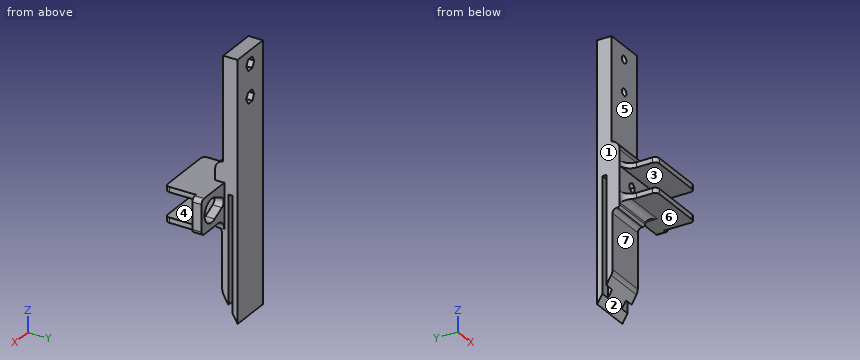
from build123d import *

# Parameters (mm, degrees)
SKETCH1_W                = 20
SKETCH1_H                = 8
BOSS_EXTRUDE1_DEPTH      = 125
CUT_EXTRUDE1_DEPTH       = 60
SKETCH3_W                = 20
SKETCH3_H                = 125
BOSS_EXTRUDE2_DEPTH      = 3
SKETCH5_W                = 4.5
SKETCH5_H                = 2
CUT_EXTRUDE2_DEPTH       = 60
BOSS_EXTRUDE5_DEPTH      = 15
BOSS_EXTRUDE5_DEPTH_BACK = 15
SKETCH9_W                = 2.5
SKETCH9_H                = 15
SKETCH10_W               = 17
SKETCH10_H               = 4.5
BOSS_EXTRUDE6_DEPTH      = 18
CUT_EXTRUDE3_DEPTH       = 129.663032374
CUT_EXTRUDE4_DEPTH       = 4
FILLET1_R                = 5
FILLET2_R                = 3
FILLET3_R                = 5
FILLET4_R                = 2
SKETCH13_W               = 46.736094472
SKETCH13_H               = 46.819354585
CUT_EXTRUDE5_DEPTH       = 30
SKETCH14_W               = 30.537207939
SKETCH14_H               = 50.61246041
CUT_EXTRUDE6_DEPTH       = 3.5
FILLET5_R                = 5
FILLET6_R                = 2
FILLET7_R                = 1
FILLET8_R                = 2
SKETCH15_W               = 20
SKETCH15_H               = 60
CUT_EXTRUDE7_DEPTH       = 5
SKETCH16_W               = 20
SKETCH16_H               = 60
BOSS_EXTRUDE7_DEPTH      = 1.5
SKETCH17_W               = 20
SKETCH17_H               = 10
BOSS_EXTRUDE8_DEPTH      = 4
FILLET9_R                = 5
SKETCH18_R               = 1.75
CUT_EXTRUDE8_DEPTH       = 131.403895283
CUT_EXTRUDE9_DEPTH       = 4


# Some blends are built 0.0001 mm under size
with BuildPart() as part:
    # Sketch1 → Boss-Extrude1 (new body)
    with BuildSketch(Plane.XY):
        with Locations((-16.536312849, 6.223463687)):
            Rectangle(SKETCH1_W, SKETCH1_H)
    extrude(amount=-BOSS_EXTRUDE1_DEPTH)

    # Sketch2 → Cut-Extrude1 (cut)
    with BuildSketch(Plane.XY):
        Polygon((-26.536312849, 7.723463687), (-22.186312849, 7.723463687), (-22.186312849, 5.723463687), (-23.686312849, 5.723463687), (-23.686312849, 4.223463687), (-22.186312849, 4.223463687), (-22.186312849, 2.723463687), (-20.536312849, 2.723463687), (-20.536312849, 7.723463687), (-12.536312849, 7.723463687), (-12.536312849, 2.723463687), (-10.886312849, 2.723463687), (-10.886312849, 4.223463687), (-9.386312849, 4.223463687), (-9.386312849, 5.723463687), (-10.886312849, 5.723463687), (-10.886312849, 7.723463687), (-6.536312849, 7.723463687), (-6.536312849, 2.223463687), (-26.536312849, 2.223463687), align=None)
    extrude(amount=-CUT_EXTRUDE1_DEPTH, mode=Mode.SUBTRACT)

    # Sketch3 → Boss-Extrude2 (add)
    with BuildSketch(Plane(origin=(0, 10.223463687, 0), x_dir=(1, 0, 0), z_dir=(0, 1, 0))):
        with Locations((-16.536312849, 62.5)):
            Rectangle(SKETCH3_W, SKETCH3_H)
    extrude(amount=BOSS_EXTRUDE2_DEPTH)

    # Sketch5 → Cut-Extrude2 (cut)
    with BuildSketch(Plane(origin=(0, 0, -125), x_dir=(-1, 0, 0), z_dir=(0, 0, -1))):
        with Locations((8.786312849, 9.723463687)):
            Rectangle(SKETCH5_W, SKETCH5_H)
        with Locations((24.286312849, 9.723463687)):
            Rectangle(SKETCH5_W, SKETCH5_H)
    extrude(amount=-CUT_EXTRUDE2_DEPTH, mode=Mode.SUBTRACT)

    # Sketch9 → Boss-Extrude5 (add, two sides: drawn at the far end of the back side and taken through both)
    with BuildSketch(Plane(origin=(-6.536312849, 0, 0), x_dir=(0, 0, -1), z_dir=(1, 0, 0)).offset(-BOSS_EXTRUDE5_DEPTH_BACK)):
        with Locations((61.25, -5.276536313)):
            Rectangle(SKETCH9_W, SKETCH9_H)
        with Locations((75.75, -5.276536313)):
            Rectangle(SKETCH9_W, SKETCH9_H)
    extrude(amount=BOSS_EXTRUDE5_DEPTH + BOSS_EXTRUDE5_DEPTH_BACK)

    # Sketch10 → Boss-Extrude6 (add)
    with BuildSketch(Plane(origin=(-6.536312849, 0, 0), x_dir=(0, 0, -1), z_dir=(1, 0, 0))):
        with Locations((68.5, 4.473463687)):
            Rectangle(SKETCH10_W, SKETCH10_H)
    extrude(amount=BOSS_EXTRUDE6_DEPTH)

    # Sketch11 → Cut-Extrude3 (cut, through all)
    with BuildSketch(Plane.XZ.offset(-2.223463687)):
        with BuildLine():
            Line((-4.650598563, -66.193892243), (1.063687151, -63.483368535))
            ThreePointArc((1.063687151, -63.483368535), (9.063687151, -68.543012791), (1.063687151, -73.602657047))
            Line((1.063687151, -73.602657047), (-4.650598563, -70.892133338))
            ThreePointArc((-4.650598563, -70.892133338), (-6.136312849, -68.543012791), (-4.650598563, -66.193892243))
        make_face()
    extrude(amount=-CUT_EXTRUDE3_DEPTH, mode=Mode.SUBTRACT)

    # Sketch12 → Cut-Extrude4 (cut)
    with BuildSketch(Plane.XZ.offset(-2.223463687)):
        Polygon((-14.717314599, -69.706805379), (-14.656689608, -67.398200185), (-16.625687858, -66.191394806), (-18.6553111, -67.293194621), (-18.71593609, -69.601799815), (-16.74693784, -70.808605194), align=None)
    extrude(amount=-CUT_EXTRUDE4_DEPTH, mode=Mode.SUBTRACT)

    # Fillet1
    fillet1_edges = [part.edges().sort_by_distance(p)[0] for p in [
        (-6.536312849, 4.473463687, -77),
    ]]
    fillet(fillet1_edges, radius=FILLET1_R)

    # Fillet2
    fillet2_edges = [part.edges().sort_by_distance(p)[0] for p in [
        (-11.536312849, 2.223463687, -77),
    ]]
    fillet(fillet2_edges, radius=FILLET2_R)

    # Fillet3
    fillet3_edges = [part.edges().sort_by_distance(p)[0] for p in [
        (-21.536312849, 2.223463687, -61.25),
        (-21.536312849, 2.223463687, -77.25),
    ]]
    fillet(fillet3_edges, radius=FILLET3_R - 0.0001)  # a hair under: the kernel refuses the full size

    # Fillet4
    fillet4_edges = [part.edges().sort_by_distance(p)[0] for p in [
        (11.463687151, 4.473463687, -77),
        (11.463687151, 4.473463687, -60),
    ]]
    fillet(fillet4_edges, radius=FILLET4_R)

    # Sketch13 → Cut-Extrude5 (cut)
    with BuildSketch(Plane(origin=(0, -44.208989971, -25.52407226), x_dir=(-1, 0, 0), z_dir=(0, 0.866025403784438, 0.500000000000001))):
        with Locations((16.217588554, -108.832455191)):
            Rectangle(SKETCH13_W, SKETCH13_H)
    extrude(amount=-CUT_EXTRUDE5_DEPTH, mode=Mode.SUBTRACT)

    # Sketch14 → Cut-Extrude6 (cut)
    with BuildSketch(Plane.XZ.offset(-2.223463687)):
        with Locations((-21.804916819, -107.306230205)):
            Rectangle(SKETCH14_W, SKETCH14_H)
    extrude(amount=-CUT_EXTRUDE6_DEPTH, mode=Mode.SUBTRACT)

    # Fillet5
    fillet5_edges = [part.edges().sort_by_distance(p)[0] for p in [
        (-16.536312849, 5.723463687, -112.009618943),
    ]]
    fillet(fillet5_edges, radius=FILLET5_R)

    # Fillet6
    fillet6_edges = [part.edges().sort_by_distance(p)[0] for p in [
        (-16.536312849, 5.723463687, -82),
    ]]
    fillet(fillet6_edges, radius=FILLET6_R)

    # Fillet7
    fillet7_edges = [part.edges().sort_by_distance(p)[0] for p in [
        (-16.536312849, 2.223463687, -82),
    ]]
    fillet(fillet7_edges, radius=FILLET7_R)

    # Fillet8
    fillet8_edges = [part.edges().sort_by_distance(p)[0] for p in [
        (-21.536312849, -12.776536313, -61.25),
        (8.463687151, -12.776536313, -61.25),
        (-21.536312849, -12.776536313, -75.75),
        (8.463687151, -12.776536313, -75.75),
    ]]
    fillet(fillet8_edges, radius=FILLET8_R)

    # Sketch15 → Cut-Extrude7 (cut)
    with BuildSketch(Plane.XZ.offset(-2.723463687)):
        with Locations((-16.536312849, -30)):
            Rectangle(SKETCH15_W, SKETCH15_H)
    extrude(amount=-CUT_EXTRUDE7_DEPTH, mode=Mode.SUBTRACT)

    # Sketch16 → Boss-Extrude7 (add)
    with BuildSketch(Plane.XZ.offset(-7.723463687)):
        with Locations((-16.536312849, -30)):
            Rectangle(SKETCH16_W, SKETCH16_H)
    extrude(amount=BOSS_EXTRUDE7_DEPTH)

    # Sketch17 → Boss-Extrude8 (add)
    with BuildSketch(Plane.XZ.offset(-6.223463687)):
        with Locations((-16.536312849, -55)):
            Rectangle(SKETCH17_W, SKETCH17_H)
    extrude(amount=BOSS_EXTRUDE8_DEPTH)

    # Fillet9
    # the kernel refuses this fillet: 5 mm, written as the material it takes off along each edge
    with BuildSketch(Plane(origin=(5.711135865, 2.223463687, -50), x_dir=(0, 1.0, -1.572075802868717e-12), z_dir=(-1, 0, 0))) as fillet9_piece_1:
        with BuildLine():
            CenterArc((5, 4.898979486), FILLET9_R, 180, 78.463040967)
            Line((0, 4.898979486), (-0.1, 4.898979486))
            Line((-0.1, 4.898979486), (-0.1, 0))
            Line((-0.1, 0), (0, -0.1))
            ThreePointArc((0, -0.1), (2, -0.1), (3.98, -0.09797959))
            Line((3.98, -0.09797959), (4, 0))
        make_face()
    extrude(amount=44.494897428, mode=Mode.SUBTRACT)

    # Sketch18 → Cut-Extrude8 (cut, through all)
    with BuildSketch(Plane(origin=(0, 13.223463687, 0), x_dir=(1, 0, 0), z_dir=(0, 1, 0))):
        with Locations(Location((-16.536312849, 22, 0), (0, 0, 270))):
            Circle(SKETCH18_R)
        with Locations(Location((-16.536312849, 6.5, 0), (0, 0, 270))):
            Circle(SKETCH18_R)
    extrude(amount=-CUT_EXTRUDE8_DEPTH, mode=Mode.SUBTRACT)

    # Sketch19 → Cut-Extrude9 (cut)
    with BuildSketch(Plane(origin=(0, 13.223463687, 0), x_dir=(1, 0, 0), z_dir=(0, 1, 0))):
        Polygon((-18.087719019, 19.224114754), (-14.908028793, 19.268500223), (-13.356622624, 22.044385468), (-14.98490668, 24.775885246), (-18.164596905, 24.731499777), (-19.716003075, 21.955614532), align=None)
        Polygon((-14.908028793, 3.768500223), (-13.356622624, 6.544385468), (-14.98490668, 9.275885246), (-18.164596905, 9.231499777), (-19.716003075, 6.455614532), (-18.087719019, 3.724114754), align=None)
    extrude(amount=-CUT_EXTRUDE9_DEPTH, mode=Mode.SUBTRACT)


solid = part.part
The listing builds one solid part. Answer for the finished solid, in the listing's coordinates (mm). Face numbers are marked on the shaded views. A direction names the side the tool comes from. Round coordinates to 2 decimals unless told otherwise and drop trailing zeros. Order: outer loops, then holes, each group sorted by start corner. A loop starts at its lowest first (then second) coordinate and runs counter-clockwise, first axis right, second up. Notation, with made-up numbers: (86, 87) -> (108, 87) arc R33 cw to (108, 123) -> close; hole circle Ø2 at (55.5, 68). An arc over 180 degrees is marked (long way). One line per item, written item: value.
Item 1: Find section C-C, the plane z = -103. Give the vertices of the cut face in (x, y), then the cut area to 3 significant figures.
Taken from the geometry:
outline: (-26.54, 5.72) -> (-6.54, 5.72) -> (-6.54, 8.72) -> (-11.04, 8.72) -> (-11.04, 10.72) -> (-6.54, 10.72) -> (-6.54, 13.22) -> (-26.54, 13.22) -> (-26.54, 10.72) -> (-22.04, 10.72) -> (-22.04, 8.72) -> (-26.54, 8.72) -> close
area: 132 mm2
Item 2: Given P1, Ø3, axis at x = -17.5, z = -69, coming from the -Y side; P2, Ø14.5, axis at x = 3, z = -66.5, coming from the +Y side; P3, Ø2, axis at x = -2, y = 3, coming from the +Z side; P4, Ø8, axis at y = 5.5, z = -19, coming from the -X side, each flat-ended and moving along its own axis, determine where each tip first touches the part or whether it passes through.
Taken from the geometry:
P1: stops at y = 2.22
P2: stops at y = 6.72
P3: stops at z = -60
P4: stops at x = -26.54
Item 3: For a pull along Z with two mould halves and no side action, classify the marked faces 1, 2, 3 and 4 as released by +Z, released by -Z, zero draft, split by the parting line, or undercut.
Taken from the geometry:
face 1: zero draft
face 2: released by -Z
face 3: undercut
face 4: undercut
Item 4: Straight lines are drawn through the part: L1, parallel to X at y = 7.7, z = -22; L2, parallel to Z at x = -2, y = -6.5; L3, parallel to Y at x = -17, z = -14. For each, find the intervals that lie inside material, in ascending order.
Taken from the geometry:
L1: x = -26.54 to -18.29, -14.79 to -6.54
L2: z = -77 to -74.5, -62.5 to -60
L3: y = 6.22 to 13.22
Item 5: Find section A-A, the plane x = 4. Give the vertices of the cut face in (y, z).
Taken from the geometry:
outline: (-12.78, -77) -> (6.72, -77) -> (6.72, -74.12) -> (2.22, -74.12) -> (2.22, -74.5) -> (-12.78, -74.5) -> close; (-12.78, -62.5) -> (2.22, -62.5) -> (2.22, -62.97) -> (6.72, -62.97) -> (6.72, -60) -> (-12.78, -60) -> close
Item 6: For the marked faces 5, 6 and 7, determine the directions among +Z, -Z, +X, -X, +Y, -Y from which every point of the face is accessible in a straight line to the end or side of a thin tool.
Taken from the geometry:
face 5: +Z, +X, -X, -Y
face 6: -Z, +X, -Y
face 7: -Z, +X, -X, -Y
Item 7: Find section D-D, the plane z = -40.5. Give the vertices of the cut face in (x, y), then the cut area to 3 significant figures.
Taken from the geometry:
outline: (-26.54, 6.22) -> (-6.54, 6.22) -> (-6.54, 13.22) -> (-26.54, 13.22) -> close
area: 140 mm2
Item 8: Find section B-B, the plane y = -6.5. Give the vertices of the cut face in (x, z), then the cut area to 3 significant figures.
Taken from the geometry:
outline: (-21.54, -77) -> (8.46, -77) -> (8.46, -74.5) -> (-21.54, -74.5) -> close; (-21.54, -62.5) -> (8.46, -62.5) -> (8.46, -60) -> (-21.54, -60) -> close
area: 150 mm2
